```python
from build123d import *

# Parameters (mm, degrees)
FILLET1_R = 0.75


with BuildPart() as part:
    # Sketch2 → Revolve1 (revolve)
    with BuildSketch(Plane(origin=(0, 0, 0), x_dir=(1, 0, 0), z_dir=(0, 1, 0))):
        Polygon((5.125, 0), (10.5, 0), (15, -15), (8.75, -15), (8.75, -11.5), (2.75, -11.5), (2.75, -10.25), (2.95, -10.25), (2.95, -10.1), (2.75, -10.1), (2.75, -3.25), (5.125, -3.25), align=None)
    revolve(axis=Axis((0, 0, 0), (0, 0, -1)))

    # Fillet1
    fillet1_edges = [part.edges().sort_by_distance(p)[0] for p in [
        (-10.5, 0, 0),
        (-15, 0, 15),
    ]]
    fillet(fillet1_edges, radius=FILLET1_R)


solid = part.part
```
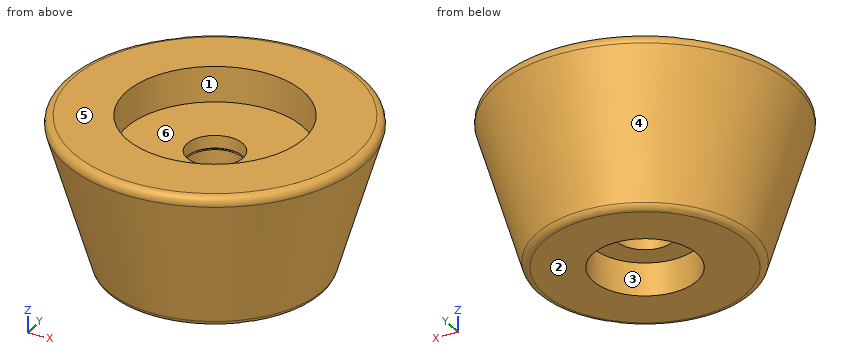
Here's how the part is built. I have some questions about the finished solid (model axes, mm). Face numbers are marked on the shaded views. A direction names the side the tool comes from. Coordinates: 2 decimals unless noted, no trailing zeros. Order: outer loops, then holes, each group sorted by start corner. A loop starts at its lowest first (then second) coordinate and runs counter-clockwise, first axis right, second up.
Item 1: If we section it at A-A, the plane x = 0: List the corners of the cut face in (y, z) for me (3 decimals), then the cut area to 3 significant figures.
Response values:
outline: (-14.71, 14.034) - (-10.66, 0.534) arc R0.75 ccw to (-9.942, 0) - (-5.125, 0) - (-5.125, 3.25) - (-2.75, 3.25) - (-2.75, 10.1) - (-2.95, 10.1) - (-2.95, 10.25) - (-2.75, 10.25) - (-2.75, 11.5) - (-8.75, 11.5) - (-8.75, 15) - (-13.992, 15) arc R0.75 ccw to start; (2.75, 3.25) - (5.125, 3.25) - (5.125, 0) - (9.942, 0) arc R0.75 ccw to (10.66, 0.534) - (14.71, 14.034) arc R0.75 ccw to (13.992, 15) - (8.75, 15) - (8.75, 11.5) - (2.75, 11.5) - (2.75, 10.25) - (2.95, 10.25) - (2.95, 10.1) - (2.75, 10.1) - close
area: 242 mm2
Item 2: I need wall thicknesses on probe 1 along Z at (x, y) = (-2.5, -1.25); probe 2 along Z at (x, y) = (2.25, -7.25); probe 3 along X at (y, z) = (0, 12.9). Which ranges of each line are inside material? Lowest first, please.
Response values:
probe 1: z = 3.25 to 10.1, 10.25 to 11.5
probe 2: z = 0 to 11.5
probe 3: x = -14.37 to -8.75, 8.75 to 14.37
Item 3: If we section it at D-D, the plane z = 9.5: List the corners of the cut face in (x, y) for me, then the cut area to 3 significant figures.
Response values:
outline: circle Ø26.7 at (0, 0); hole circle Ø5.5 at (0, 0)
area: 536 mm2
Item 4: Thinking about a two-plate mould opening in X: for the marked faces 1, 2, 3 and 4, which applies, pulls with the +X half, pulls with the -X half, needs draft (parallel to the pull), parting line crosses it, or undercut?
Response values:
face 1: undercut
face 2: needs draft
face 3: undercut
face 4: parting line crosses it
Item 5: Which directions (+Z, -Z, +X, -X, +Y, -Y) give clear straight access to the entire face, cutting with the end or side of a thin tool? Please do the marked faces 5 and 6.
Response values:
face 5: +Z, +X, -X, +Y, -Y
face 6: +Z
Item 6: If we section it at C-C, the plane z = 5: List the corners of the cut face in (x, y) for me.
Response values:
outline: circle Ø24 at (0, 0); hole circle Ø5.5 at (0, 0)
Item 7: I'm going to push flat-ended pins straight in: pin 1 Ø6 at (x, z) = (8.5, 3.5) entering from +Y; pin 2 Ø3 at (x, y) = (-1.5, 0.5) entering from -Z; pin 3 Ø1 at (y, z) = (9, 10) entering from -X. Where does each tip first touch, or does it pass through?
Response values:
pin 1: stops at y = 10.45
pin 2: stops at z = 3.25
pin 3: stops at x = -10.53
